Can you work these out from the model? Positions are in its coordinate system, mm. Give positions to 0.01 mm unless a question says otherwise; leave off trailing zeros. Answer as a JSON object with one key per item and string values.
```python
from build123d import *

# Parameters (mm, degrees)
F0_W     = 222.25
F0_H     = 146.05
F1_DEPTH = 9.525
F2_W     = 69.85
F2_H     = 38.1
F2_H_2   = 133.35
F2_H_3   = 31.75
F2_W_2   = 44.45
F2_H_4   = 60.325
F3_DEPTH = 6.35
F4_F1_R  = 6.35
F4_F2_R  = 6.35
F4_F3_R  = 6.35
F4_F4_R  = 6.35
F4_F5_R  = 6.35
F4_F6_R  = 6.3499
F4_F7_R  = 6.35
F4_F8_R  = 6.3499
F4_F9_R  = 6.35
F4_F10_R = 6.35
F4_F11_R = 6.3499
F4_F12_R = 6.3499
F4_F13_R = 6.35
F4_F14_R = 6.3499
F4_F15_R = 6.3499
F4_F16_R = 6.3499
F4_F17_R = 6.35
F4_F18_R = 6.35
F4_F19_R = 6.3499
F4_F20_R = 6.3499
F4_F21_R = 6.35
F4_F22_R = 6.3499
F4_F23_R = 6.3499
F4_F24_R = 6.3499
F4_F25_R = 6.35
F4_F26_R = 6.35
F4_F27_R = 6.3499
F4_F28_R = 6.3499


# Not quite as in the source:
# - two fillets or chamfers of one size are made in one step
# - a fillet or chamfer is up to 0.001 mm smaller than in the source, because OpenCascade refuses the exact size
# - a feature of the source that left no trace in its solid (it failed there, or was rolled back) is left out


with BuildPart() as f1:
    # F0 (on Top) → F1 (new body)
    with BuildSketch(Plane.XY):
        Rectangle(F0_W, F0_H)
    extrude(amount=F1_DEPTH)

    # F2 (on face) → F3 (cut)
    with BuildSketch(Plane.XY.offset(9.525)):
        with Locations((69.85, 47.625)):
            Rectangle(F2_W, F2_H)
        with Locations((69.85, -47.625)):
            Rectangle(F2_W, F2_H)
        with Locations((-69.85, 0)):
            Rectangle(F2_W, F2_H_2)
        with Locations((69.85, 0)):
            Rectangle(F2_W, F2_H_3)
        with Locations((0, -36.5125)):
            Rectangle(F2_W_2, F2_H_4)
        with Locations((0, 36.5125)):
            Rectangle(F2_W_2, F2_H_4)
    extrude(amount=-F3_DEPTH, mode=Mode.SUBTRACT)

    # F4: fillet of radius 6.35 on 46 edges, made by hand

    # F4_f1
    f4_f1_edges = [f1.edges().sort_by_distance(p)[0] for p in [
        (111.125, -73.025, 4.7625),
    ]]
    fillet(f4_f1_edges, radius=F4_F1_R)

    # F4_f2
    f4_f2_edges = [f1.edges().sort_by_distance(p)[0] for p in [
        (111.125, 73.025, 4.7625),
    ]]
    fillet(f4_f2_edges, radius=F4_F2_R)

    # F4_f3
    f4_f3_edges = [f1.edges().sort_by_distance(p)[0] for p in [
        (-111.125, -73.025, 4.7625),
    ]]
    fillet(f4_f3_edges, radius=F4_F3_R)

    # F4_f4
    f4_f4_edges = [f1.edges().sort_by_distance(p)[0] for p in [
        (-111.125, 73.025, 4.7625),
    ]]
    fillet(f4_f4_edges, radius=F4_F4_R)

    # F4_f5
    f4_f5_edges = [f1.edges().sort_by_distance(p)[0] for p in [
        (-22.225, -6.35, 6.35),
    ]]
    fillet(f4_f5_edges, radius=F4_F5_R)

    # F4_f6 (radius 6.35 in the source; OpenCascade refuses exactly that, so slightly less here)
    f4_f6_edges = [f1.edges().sort_by_distance(p)[0] for p in [
        (-22.225, -39.6875, 3.175),
    ]]
    fillet(f4_f6_edges, radius=F4_F6_R)

    # F4_f7
    f4_f7_edges = [f1.edges().sort_by_distance(p)[0] for p in [
        (22.225, -66.675, 6.35),
    ]]
    fillet(f4_f7_edges, radius=F4_F7_R)

    # F4_f8 (radius 6.35 in the source; OpenCascade refuses exactly that, so slightly less here)
    f4_f8_edges = [f1.edges().sort_by_distance(p)[0] for p in [
        (-5e-05, -66.675, 3.175),
    ]]
    fillet(f4_f8_edges, radius=F4_F8_R)

    # F4_f9
    f4_f9_edges = [f1.edges().sort_by_distance(p)[0] for p in [
        (34.925, -66.675, 6.35),
    ]]
    fillet(f4_f9_edges, radius=F4_F9_R)

    # F4_f10
    f4_f10_edges = [f1.edges().sort_by_distance(p)[0] for p in [
        (104.775, -66.675, 6.35),
    ]]
    fillet(f4_f10_edges, radius=F4_F10_R)

    # F4_f11 (radius 6.35 in the source; OpenCascade refuses exactly that, so slightly less here)
    f4_f11_edges = [f1.edges().sort_by_distance(p)[0] for p in [
        (69.85, -66.675, 3.175),
    ]]
    fillet(f4_f11_edges, radius=F4_F11_R)

    # F4_f12 (radius 6.35 in the source; OpenCascade refuses exactly that, so slightly less here)
    f4_f12_edges = [f1.edges().sort_by_distance(p)[0] for p in [
        (104.775, -28.575, 9.52495),
    ]]
    fillet(f4_f12_edges, radius=F4_F12_R)

    # F4_f13
    f4_f13_edges = [f1.edges().sort_by_distance(p)[0] for p in [
        (-34.925, 66.675, 6.35),
    ]]
    fillet(f4_f13_edges, radius=F4_F13_R)

    # F4_f14 (radius 6.35 in the source; OpenCascade refuses exactly that, so slightly less here)
    f4_f14_edges = [f1.edges().sort_by_distance(p)[0] for p in [
        (-73.025, 66.675, 3.175),
    ]]
    fillet(f4_f14_edges, radius=F4_F14_R)

    # F4_f15 (radius 6.35 in the source; OpenCascade refuses exactly that, so slightly less here)
    f4_f15_edges = [f1.edges().sort_by_distance(p)[0] for p in [
        (-104.775, -3.17495, 3.175),
    ]]
    fillet(f4_f15_edges, radius=F4_F15_R)

    # F4_f16 (radius 6.35 in the source; OpenCascade refuses exactly that, so slightly less here)
    f4_f16_edges = [f1.edges().sort_by_distance(p)[0] for p in [
        (-34.925, -66.675, 9.52495),
    ]]
    fillet(f4_f16_edges, radius=F4_F16_R)

    # F4_f17
    f4_f17_edges = [f1.edges().sort_by_distance(p)[0] for p in [
        (104.775, -15.875, 6.35),
    ]]
    fillet(f4_f17_edges, radius=F4_F17_R)

    # F4_f18
    f4_f18_edges = [f1.edges().sort_by_distance(p)[0] for p in [
        (104.775, 15.875, 6.35),
    ]]
    fillet(f4_f18_edges, radius=F4_F18_R)

    # F4_f19 (radius 6.35 in the source; OpenCascade refuses exactly that, so slightly less here)
    f4_f19_edges = [f1.edges().sort_by_distance(p)[0] for p in [
        (104.775, 0, 3.175),
    ]]
    fillet(f4_f19_edges, radius=F4_F19_R)

    # F4_f20 (radius 6.35 in the source; OpenCascade refuses exactly that, so slightly less here)
    f4_f20_edges = [f1.edges().sort_by_distance(p)[0] for p in [
        (34.925, 15.875, 9.52495),
    ]]
    fillet(f4_f20_edges, radius=F4_F20_R)

    # F4_f21
    f4_f21_edges = [f1.edges().sort_by_distance(p)[0] for p in [
        (22.225, 6.35, 6.35),
    ]]
    fillet(f4_f21_edges, radius=F4_F21_R)

    # F4_f22 (radius 6.35 in the source; OpenCascade refuses exactly that, so slightly less here)
    f4_f22_edges = [f1.edges().sort_by_distance(p)[0] for p in [
        (22.225, 39.6875, 3.175),
    ]]
    fillet(f4_f22_edges, radius=F4_F22_R)

    # F4_f23 (radius 6.35 in the source; OpenCascade refuses exactly that, so slightly less here)
    f4_f23_edges = [f1.edges().sort_by_distance(p)[0] for p in [
        (-3.17495, 66.675, 3.175),
    ]]
    fillet(f4_f23_edges, radius=F4_F23_R)

    # F4_f24 (radius 6.35 in the source; OpenCascade refuses exactly that, so slightly less here)
    f4_f24_edges = [f1.edges().sort_by_distance(p)[0] for p in [
        (-22.225, 6.35, 9.52495),
    ]]
    fillet(f4_f24_edges, radius=F4_F24_R)

    # F4_f25
    f4_f25_edges = [f1.edges().sort_by_distance(p)[0] for p in [
        (104.775, 28.575, 6.35),
    ]]
    fillet(f4_f25_edges, radius=F4_F25_R)

    # F4_f26
    f4_f26_edges = [f1.edges().sort_by_distance(p)[0] for p in [
        (104.775, 66.675, 6.35),
    ]]
    fillet(f4_f26_edges, radius=F4_F26_R)

    # F4_f27 (radius 6.35 in the source; OpenCascade refuses exactly that, so slightly less here)
    f4_f27_edges = [f1.edges().sort_by_distance(p)[0] for p in [
        (104.775, 47.625, 3.175),
    ]]
    fillet(f4_f27_edges, radius=F4_F27_R)

    # F4_f28 (radius 6.35 in the source; OpenCascade refuses exactly that, so slightly less here)
    f4_f28_edges = [f1.edges().sort_by_distance(p)[0] for p in [
        (34.925, 66.675, 9.52495),
    ]]
    fillet(f4_f28_edges, radius=F4_F28_R)


solid = f1.part
```
1) Imagine slicing it at C-C on z = 7. Give the number of separate pieces and of enclosed holes in the cut face, and give its area (3 significant figures).
Check sheet entries:
{"separate pieces": "1", "enclosed holes": "6", "area": "11,100 mm2"}
2) If we mould it in two halves opening along X, with no side actions, what happens to faces 1 (the cylindrical face through (-109.31, 71.12, 4.83)), 2 (the flat face through (16, 0, 9.525)), 3 (the flat face through (69, 0, 3.175))? For each: released by +X, released by -X, zero draft, split by the parting line, or undercut.
Check sheet entries:
{"face 1": "released by -X", "face 2": "zero draft", "face 3": "undercut"}
3) I need wall thicknesses on L1, parallel to X at y = 6, z = 9.25 (3 decimals); L2, parallel to Y at x = 41, z = 8.5 (3 decimals); L3, parallel to Y at x = -15.5, z = 6.25 (3 decimals). Which ranges of each line are inside material? Lowest first, please.
Check sheet entries:
{"L1": "-111.125 to -104.769, -34.931 to 34.931, 104.769 to 111.125", "L2": "-73.025 to -66.586, -28.664 to -15.786, 15.786 to 28.664, 66.586 to 73.025", "L3": "-73.025 to -65.765, -7.26 to 7.26, 65.765 to 73.025"}
4) I'm going to push a flat-ended pin straight in: P1, Ø10, axis at x = -81.5, y = 13, coming from the +Z side (3 decimals). Where does the tip first touch, or does it pass through?
Check sheet entries:
{"P1": "z = 3.175"}
